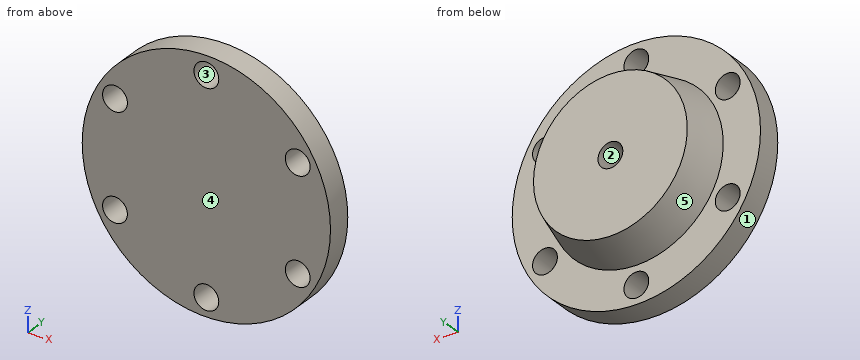
```python
from build123d import *

# Parameters (mm, degrees)
SKETCH2_R           = 254
SKETCH2_R_2         = 25.4
BOSS_EXTRUDE2_DEPTH = 50.8
SKETCH3_R           = 177.8
BOSS_EXTRUDE3_DEPTH = 76.2
BOSS_EXTRUDE3_TAPER = 15
SKETCH4_R           = 25.4
CUT_EXTRUDE1_DEPTH  = 76.2


with BuildPart() as part:
    # Sketch2 → Boss-Extrude2 (new body)
    with BuildSketch(Plane(origin=(0, 0, 0), x_dir=(1, 0, 0), z_dir=(0, 1, 0))):
        Circle(SKETCH2_R)
        with Locations((0, 215.9)):
            Circle(SKETCH2_R_2, mode=Mode.SUBTRACT)
        with Locations((186.974884677, 107.95)):
            Circle(SKETCH2_R_2, mode=Mode.SUBTRACT)
        with Locations((186.974884677, -107.95)):
            Circle(SKETCH2_R_2, mode=Mode.SUBTRACT)
        with Locations((0, -215.9)):
            Circle(SKETCH2_R_2, mode=Mode.SUBTRACT)
        with Locations((-186.974884677, -107.95)):
            Circle(SKETCH2_R_2, mode=Mode.SUBTRACT)
        with Locations((-186.974884677, 107.95)):
            Circle(SKETCH2_R_2, mode=Mode.SUBTRACT)
    extrude(amount=BOSS_EXTRUDE2_DEPTH)

    # Sketch3 → Boss-Extrude3 (add)
    with BuildSketch(Plane(origin=(0, 50.8, 0), x_dir=(1, 0, 0), z_dir=(0, 1, 0))):
        Circle(SKETCH3_R)
    extrude(amount=BOSS_EXTRUDE3_DEPTH, taper=BOSS_EXTRUDE3_TAPER)

    # Sketch4 → Cut-Extrude1 (cut)
    with BuildSketch(Plane(origin=(0, 127, 0), x_dir=(1, 0, 0), z_dir=(0, 1, 0))):
        Circle(SKETCH4_R)
    extrude(amount=-CUT_EXTRUDE1_DEPTH, mode=Mode.SUBTRACT)


solid = part.part
```
Build history of the part. All positions in model axes, mm. Face numbers are marked on the shaded views. A direction names the side the tool comes from. Round coordinates to 2 decimals unless told otherwise and drop trailing zeros. Order: outer loops, then holes, each group sorted by start corner. A loop starts at its lowest first (then second) coordinate and runs counter-clockwise, first axis right, second up. Notation, with made-up numbers: (22, -19) - (55, -19) arc R31 cw to (55, 10) - close; hole circle Ø2 at (10.25, 89.5). An arc over 180 degrees is marked (long way). Use a Markdown table: item, result.
1) Flat gauge pins, fed straight in: pin 1 Ø12 at (y, z) = (79, 24.5) entering from -X; pin 2 Ø1.5 at (x, y) = (48, 107) entering from -Z; pin 3 Ø15 at (x, z) = (-8.5, 8.5) entering from +Y. Where does each tip first touch, or does it go through?
Recorded:
| item | result |
|---|---|
| pin 1 | stops at x = -170.29 |
| pin 2 | stops at z = -155.81 |
| pin 3 | stops at y = 50.8 |
2) Saw through at B-B on y = 8.5. Write the cut outline in (x, z).
Recorded:
| item | result |
|---|---|
| outline | circle Ø508 at (0, 0); hole circle Ø50.8 at (-186.97, -107.95); hole circle Ø50.8 at (-186.97, 107.95); hole circle Ø50.8 at (0, -215.9); hole circle Ø50.8 at (0, 215.9); hole circle Ø50.8 at (186.97, -107.95); hole circle Ø50.8 at (186.97, 107.95) |
3) Saw through at C-C on z = 215.9. Write the cut outline in (x, y).
Recorded:
| item | result |
|---|---|
| outline | (-133.8, 0) - (-25.4, 0) - (-25.4, 50.8) - (-133.8, 50.8) - close; (25.4, 0) - (133.8, 0) - (133.8, 50.8) - (25.4, 50.8) - close |
4) Saw through at D-D on z = 107.95. Give the number of separate pieces and of enclosed holes in the cut face, and give its area (3 significant figures).
Recorded:
| item | result |
|---|---|
| separate pieces | 3 |
| enclosed holes | 0 |
| area | 37,700 mm² |
5) Saw through at A-A on x = 0. Write the cut outline in (y, z), and give its area (3 significant figures).
Recorded:
| item | result |
|---|---|
| outline | (0, -254) - (50.8, -254) - (50.8, -241.3) - (0, -241.3) - close; (0, -190.5) - (50.8, -190.5) - (50.8, -177.8) - (127, -157.38) - (127, -25.4) - (50.8, -25.4) - (50.8, 25.4) - (127, 25.4) - (127, 157.38) - (50.8, 177.8) - (50.8, 190.5) - (0, 190.5) - close; (0, 241.3) - (50.8, 241.3) - (50.8, 254) - (0, 254) - close |
| area | 42,300 mm² |
6) Tool access for the marked faces 1 and 2: list every direction of +Z, -Z, +X, -X, +Y, -Y with a clear straight run to the whole face (end or side of a thin tool).
Recorded:
| item | result |
|---|---|
| face 1 | +Y, -Y |
| face 2 | +Y |
7) Wall check: L1, parallel to Z at x = 0, y = 40; L2, parallel to Z at x = -206.5, y = 21.5; L3, parallel to X at y = 18, z = 107. Give the ranges that are in metal, low to high.
Recorded:
| item | result |
|---|---|
| L1 | z = -254 to -241.3, -190.5 to 190.5, 241.3 to 254 |
| L2 | z = -147.9 to -124.2, -91.7 to 91.7, 124.2 to 147.9 |
| L3 | x = -230.36 to -212.36, -161.59 to 161.59, 212.36 to 230.36 |
8) Pull direction Z, two halves, no side cores. Call the marked faces 3, 4 and 5: pulls with the +Z half, pulls with the -Z half, needs draft (parallel to the pull), parting line crosses it, or undercut.
Recorded:
| item | result |
|---|---|
| face 3 | undercut |
| face 4 | needs draft |
| face 5 | parting line crosses it |
